```python
from build123d import *

# Parameters (mm, degrees)
SKETCH_1_R             = 30
EXTRUDE_1_DEPTH        = 5
SKETCH_2_R             = 35
SKETCH_2_R_2           = 30
EXTRUDE_2_DEPTH        = 1
SKETCH_4_R             = 42.5
SKETCH_4_R_2           = 35
EXTRUDE_3_DEPTH        = 2
SKETCH_5_R             = 2
CUT_EXTRUDE_3_DEPTH    = 61.51033
SKETCH_6_R             = 10
EXTRUDE_4_DEPTH        = 5
FILLET_1_R             = 2
FILLET_1_OF_MIRROR_1_R = 2
EXTRUDE_5_DEPTH        = 5


with BuildPart() as part:
    # 草图1 → 凸台-拉伸1 (new body)
    with BuildSketch(Plane.XY):
        with BuildLine():
            Line((-30.103986, -30), (-40, -30))
            Line((-40, -30), (-40, 30))
            Line((-40, 30), (-30.103986, 30))
            ThreePointArc((-30.103986, 30), (0, 42.5), (30.103986, 30))
            Line((30.103986, 30), (40, 30))
            Line((40, 30), (40, -30))
            Line((40, -30), (30.103986, -30))
            ThreePointArc((30.103986, -30), (0, -42.5), (-30.103986, -30))
        make_face()
        Circle(SKETCH_1_R, mode=Mode.SUBTRACT)
    extrude(amount=EXTRUDE_1_DEPTH)

    # 草图2 → 凸台-拉伸2 (add)
    with BuildSketch(Plane.XY.offset(5)):
        Circle(SKETCH_2_R)
        Circle(SKETCH_2_R_2, mode=Mode.SUBTRACT)
    extrude(amount=EXTRUDE_2_DEPTH)

    # 草图4 → 凸台-拉伸3 (add)
    with BuildSketch(Plane.XY.offset(5)):
        with Locations(Location((0, 0, 0), (0, 0, 160.250077))):
            Circle(SKETCH_4_R)
        Circle(SKETCH_4_R_2, mode=Mode.SUBTRACT)
    extrude(amount=EXTRUDE_3_DEPTH)

    # 草图5 → 切除-拉伸3 (cut, through all)
    with BuildSketch(Plane(origin=(0, 0, 0), x_dir=(-1, 0, 0), z_dir=(0, 0, -1))):
        with Locations((0, 35)):
            Circle(SKETCH_5_R)
        with Locations((35, 0)):
            Circle(SKETCH_5_R)
        with Locations((0, -35)):
            Circle(SKETCH_5_R)
        with Locations((-35, 0)):
            Circle(SKETCH_5_R)
    extrude(amount=-CUT_EXTRUDE_3_DEPTH, mode=Mode.SUBTRACT)

    # 草图6 → 凸台-拉伸4 (add)
    with BuildSketch(Plane.ZY.offset(40)):
        with BuildLine():
            Line((5, -30), (-35, -30))
            ThreePointArc((-35, -30), (-65, 0), (-35, 30))
            Line((-35, 30), (5, 30))
            Line((5, 30), (5, -30))
        make_face()
        with Locations((-35, 0)):
            Circle(SKETCH_6_R, mode=Mode.SUBTRACT)
    extrude_4 = extrude(amount=EXTRUDE_4_DEPTH)

    # 圆角1
    fillet_1_edges = [part.edges().sort_by_distance(p)[0] for p in [
        (-45, 0, 5),
    ]]
    fillet(fillet_1_edges, radius=FILLET_1_R)

    # 镜向1: 凸台-拉伸4 across plane
    add(extrude_4.mirror(Plane(origin=(0, 0, 0), x_dir=(0, 0, 1), z_dir=(1, 0, 0))))

    # 圆角1 of 镜向1
    fillet_1_of_mirror_1_edges = [part.edges().sort_by_distance(p)[0] for p in [
        (45, 0, 5),
    ]]
    fillet(fillet_1_of_mirror_1_edges, radius=FILLET_1_OF_MIRROR_1_R)

    # 草图7 → 凸台-拉伸5 (add)
    with BuildSketch(Plane(origin=(0, 0, 0), x_dir=(-1, 0, 0), z_dir=(0, 0, -1))):
        with BuildLine():
            Line((-8, -6), (-29.686217, -6))
            ThreePointArc((-29.686217, -6), (-30.28649, 0), (-29.686217, 6))
            Line((-29.686217, 6), (-8, 6))
            ThreePointArc((-8, 6), (10, 0), (-8, -6))
        make_face()
    extrude(amount=-EXTRUDE_5_DEPTH)


solid = part.part
```
Verification items for the finished model (mm, model axes). A direction names the side the tool comes from. Round coordinates to 2 decimals unless told otherwise and drop trailing zeros. Order: outer loops, then holes, each group sorted by start corner. A loop starts at its lowest first (then second) coordinate and runs counter-clockwise, first axis right, second up.
1) Material ranges on line 1 (Y direction, x = 0, z = 2.75); line 2 (X direction, y = 0, z = 5.75); line 3 (X direction, y = 24.5, z = -29), recorded low to high.
Geometry says:
line 1: y = -42.5 to -37, -33 to -30, -10 to 10, 30 to 33, 37 to 42.5
line 2: x = -42.5 to -37, -33 to -30, 30 to 33, 37 to 42.5
line 3: x = -45 to -40, 40 to 45
2) Cross-section at D-D, the plane z = -38.5. Record the cut outline in (x, y), plus the area to 3 significant figures.
Geometry says:
outline: (-45, -29.8) - (-40, -29.8) - (-40, -9.37) - (-45, -9.37) - close; (-45, 9.37) - (-40, 9.37) - (-40, 29.8) - (-45, 29.8) - close; (40, -29.8) - (45, -29.8) - (45, -9.37) - (40, -9.37) - close; (40, 9.37) - (45, 9.37) - (45, 29.8) - (40, 29.8) - close
area: 409 mm2
3) Draft check along Z on faces 6 (the cylindrical face through (-25, -24.495, 6.493)), 7 (the cylindrical face through (-42.465, -0.66, -64.993)), 8 (the flat face through (-6, -35, 7)), 9 (the cylindrical face through (-42, 0, -45)). Enter one of: +Z half, -Z half, draft (parallel to the pull), parting line (faces both ways), or undercut.
Geometry says:
face 6: draft
face 7: -Z half
face 8: +Z half
face 9: undercut
4) Depth check by flat-ended pin: pin 1 (6 mm diameter, centred on x = 24.5, z = -1.5, fed in from -Y); pin 2 (24 mm diameter, centred on x = 18.5, y = -6.5, fed in from -Z); pin 3 (5.5 mm diameter, centred on x = 17, z = 3.5, fed in from +Y); pin 4 (2.5 mm diameter, centred on x = 0, y = 35, fed in from +Z). Enter the tip coordinate at first touch or a pass-through.
Geometry says:
pin 1: stops at y = -36.42
pin 2: stops at z = 0
pin 3: stops at y = 40.04
pin 4: passes through
5) Cross-section at C-C, the plane y = -21. Record the cut outline in (x, z), plus the area to 3 significant figures.
Geometry says:
outline: (-45, -56.42) - (-40, -56.42) - (-40, 0) - (-21.42, 0) - (-21.42, 6) - (-28, 6) - (-28, 7) - (-36.95, 7) - (-36.95, 5) - (-43, 5) arc R2 ccw to (-45, 3) - close; (21.42, 0) - (40, 0) - (40, -56.42) - (45, -56.42) - (45, 3) arc R2 ccw to (43, 5) - (36.95, 5) - (36.95, 7) - (28, 7) - (28, 6) - (21.42, 6) - close
area: 847 mm2
6) Cross-section at A-A, the plane z = -21.5. Record the cut outline in (x, y), plus the area to 3 significant figures.
Geometry says:
outline: (-45, -30) - (-40, -30) - (-40, 30) - (-45, 30) - close; (40, -30) - (45, -30) - (45, 30) - (40, 30) - close
area: 600 mm2
7) Cross-section at B-B, the plane x = 0. Record the cut outline in (y, z).
Geometry says:
outline: (-42.5, 0) - (-37, 0) - (-37, 7) - (-42.5, 7) - close; (-33, 0) - (-30, 0) - (-30, 6) - (-33, 6) - close; (-10, 0) - (10, 0) - (10, 5) - (-10, 5) - close; (30, 0) - (33, 0) - (33, 6) - (30, 6) - close; (37, 0) - (42.5, 0) - (42.5, 7) - (37, 7) - close
8) Tool access check on faces 1 (the flat face through (42.7, -2.1, 5)), 2 (the flat face through (-42.7, -2.1, 5)), 3 (the flat face through (-1, 1, 0)), 4 (the flat face through (41, -30, -10)), 5 (the flat face through (15.4, 26, 6)). Record the directions out of +Z, -Z, +X, -X, +Y, -Y that give a thin tool (end or side, any length) a straight path to the whole face; none if there is none.
Geometry says:
face 1: +Z, +X
face 2: +Z, -X
face 3: -Z, +Y, -Y
face 4: +Z, -Z, +X, -Y
face 5: +Z
